```python
from build123d import *

# Parameters (mm, degrees)
SKETCH2_W           = 35
SKETCH2_H           = 30
BOSS_EXTRUDE1_DEPTH = 18
SKETCH3_R           = 1.7
CUT_EXTRUDE1_DEPTH  = 50.487372127
SKETCH4_R           = 4
CUT_EXTRUDE2_DEPTH  = 50.487372127


with BuildPart() as part:
    # Sketch2 → Boss-Extrude1 (new body)
    with BuildSketch(Plane(origin=(0, 0, 0), x_dir=(1, 0, 0), z_dir=(0, 1, 0))):
        with Locations((17.5, 15)):
            Rectangle(SKETCH2_W, SKETCH2_H)
    extrude(amount=BOSS_EXTRUDE1_DEPTH)

    # Sketch3 → Cut-Extrude1 (cut, through all)
    with BuildSketch(Plane.XZ):
        with Locations(Location((5.5, -24, 0), (0, 0, 270))):
            Circle(SKETCH3_R)
        with Locations(Location((29.5, -24, 0), (0, 0, 90))):
            Circle(SKETCH3_R)
        with Locations(Location((29.5, -6, 0), (0, 0, 270))):
            Circle(SKETCH3_R)
        with Locations(Location((5.5, -6, 0), (0, 0, 90))):
            Circle(SKETCH3_R)
    extrude(amount=-CUT_EXTRUDE1_DEPTH, mode=Mode.SUBTRACT)

    # Sketch4 → Cut-Extrude2 (cut, through all)
    with BuildSketch(Plane.XY):
        with Locations((17.5, 8)):
            Circle(SKETCH4_R)
    extrude(amount=-CUT_EXTRUDE2_DEPTH, mode=Mode.SUBTRACT)


solid = part.part
```
Here's how the part is built. I have some questions about the finished solid (model axes, mm). Round coordinates to 2 decimals unless told otherwise and drop trailing zeros. Order: outer loops, then holes, each group sorted by start corner. A loop starts at its lowest first (then second) coordinate and runs counter-clockwise, first axis right, second up. Notation, with made-up numbers: M 33.25,46.25 L 65.25,46.25 A17 ccw 65.25,79.25 Z; hole C -33.5,-20 d1. An arc over 180 degrees is marked long. Answer in a Markdown table with one row per item.
Item 1: Imagine slicing it at D-D, the plane x = 5.5. Write out the boundary of the cut face in (y, z), and give its area (3 significant figures).
A:
| item | result |
|---|---|
| outline | M 0,-30 L 18,-30 L 18,-25.7 L 0,-25.7 Z; M 0,-22.3 L 18,-22.3 L 18,-7.7 L 0,-7.7 Z; M 0,-4.3 L 18,-4.3 L 18,0 L 0,0 Z |
| area | 418 mm2 |
Item 2: If I drill on L1, parallel to X at y = 13.75, z = -6; L2, parallel to Z at x = 6, y = 1.5; L3, parallel to X at y = 7.5, z = -23.5, over which ranges is the centre line in solid material (lowest first)? Write a range as from..to.
A:
| item | result |
|---|---|
| L1 | x = 0..3.8, 7.2..27.8, 31.2..35 |
| L2 | z = -30..-25.62, -22.38..-7.62, -4.38..0 |
| L3 | x = 0..3.88, 7.12..13.53, 21.47..27.88, 31.12..35 |
Item 3: Imagine slicing it at B-B, the plane y = 8. Write out the boundary of the cut face in (x, z), and give its area (3 significant figures).
A:
| item | result |
|---|---|
| outline | M 0,-30 L 13.5,-30 L 13.5,0 L 0,0 Z; M 21.5,-30 L 35,-30 L 35,0 L 21.5,0 Z; hole C 5.5,-24 d3.4; hole C 5.5,-6 d3.4; hole C 29.5,-24 d3.4; hole C 29.5,-6 d3.4 |
| area | 774 mm2 |
Item 4: Imagine slicing it at A-A, the plane z = -24. Write out the boundary of the cut face in (x, y).
A:
| item | result |
|---|---|
| outline | M 0,0 L 3.8,0 L 3.8,18 L 0,18 Z; M 7.2,0 L 27.8,0 L 27.8,18 L 7.2,18 Z; M 31.2,0 L 35,0 L 35,18 L 31.2,18 Z; hole C 17.5,8 d8 |
Item 5: Thinking about a two-plate mould opening in Z: for faces 1 (the face through (7.16, 8.87, -6.37)), 2 (the face through (13, 9, -30)), 3 (the face through (0, 9, -15)), which applies, +Z half, -Z half, draft (parallel to the pull), parting line (faces both ways), or undercut?
A:
| item | result |
|---|---|
| face 1 | undercut |
| face 2 | -Z half |
| face 3 | draft |
Item 6: Imagine slicing it at C-C, the plane x = 17.5. Write out the boundary of the cut face in (y, z).
A:
| item | result |
|---|---|
| outline | M 0,-30 L 4,-30 L 4,0 L 0,0 Z; M 12,-30 L 18,-30 L 18,0 L 12,0 Z |
